```python
from build123d import *

# Parameters (mm, degrees)
F0_W     = 55.499
F0_H     = 37.5412
F0_W_2   = 52.959
F0_H_2   = 35.0012
F1_DEPTH = 1.27
F2_DEPTH = 7.62
F3_R     = 10.16


with BuildPart() as f1:
    # F0 (on Top) → F1 (new body)
    with BuildSketch(Plane.XY):
        with Locations((-37.199277, 3.972059)):
            Rectangle(F0_W, F0_H)
        with Locations((-37.199277, 3.972059)):
            Rectangle(F0_W_2, F0_H_2, mode=Mode.SUBTRACT)
        with Locations((-37.199277, 3.972059)):
            Rectangle(F0_W_2, F0_H_2)
    extrude(amount=F1_DEPTH)

    # F0 (on Top) → F2 (join)
    with BuildSketch(Plane.XY):
        with Locations((-37.199277, 3.972059)):
            Rectangle(F0_W, F0_H)
        with Locations((-37.199277, 3.972059)):
            Rectangle(F0_W_2, F0_H_2, mode=Mode.SUBTRACT)
    extrude(amount=F2_DEPTH)

    # F3
    f3_edges = [f1.edges().sort_by_distance(p)[0] for p in [
        (-64.948777, 22.742659, 3.81),
        (-63.678777, 21.472659, 4.445),
        (-10.719777, -13.528541, 4.445),
        (-9.449777, -14.798541, 3.81),
    ]]
    fillet(f3_edges, radius=F3_R)


solid = f1.part
```
The listing builds one solid part. Answer for the finished solid, in the listing's coordinates (mm). A direction names the side the tool comes from. Coordinates: 2 decimals unless noted, no trailing zeros. Loops run counter-clockwise (first coordinate to the right, second up) from the corner with the lowest first, then second, coordinate; pieces in that order, holes last. Notation, with made-up numbers: (81, 45) -> (121, 45) arc R28 cw to (121, 80) -> close; hole circle Ø8 at (78.5, -17). An arc over 180 degrees is marked (long way). Return JSON: item names as keys, results as strings. Group by question number.
(1) A cutting plane is placed at A-A on z = 3.5. Write down the section's boundary in (x, y).
(2) A cutting plane is placed at C-C on y = 9. Write down the section's boundary in (x, z), and give its area (3 significant figures).
(3) Given pin 1 Ø2 at (x, z) = (-18, 3.5) entering from -Y; pin 2 Ø10 at (x, y) = (-32.5, 16) entering from +Z, each flat-ended and moving along its own axis, determine where each tip first touches the part or whether it passes through.
(4) A cutting plane is placed at B-B on x = -44. Write down the section's boundary in (y, z).
(5) Determine the mould class of faces 3 (the flat face through (-64.949, -1, 4)), 4 (the flat face through (-10.72, 9, 4)), 5 (the flat face through (-43, -14.799, 4)), 6 (the flat face through (-9.45, 9, 4)) for opening direction X: released by +X, released by -X, zero draft, split by the parting line, or undercut.
(6) Find the intervals of material crossed by probe 1 along Y at (x, z) = (-32.5, 2.5); probe 2 along X at (y, z) = (2.5, 1.5); probe 3 along Z at (x, y) = (-13, 19.5), in increasing order. Write a range as from..to.
(7) Which of the six approach directions +Z, -Z, +X, -X, +Y, -Y give full straight-line access (tool end or side, diameter ignored) to faces 1 (the flat face through (-43, -13.529, 4)), 2 (the cylindrical face through (-12.347, -11.743, 3.863))?
The answers:
{
 "1": {"outline": "(-64.95, -14.8) -> (-19.61, -14.8) arc R10.16 ccw to (-9.45, -4.64) -> (-9.45, 22.74) -> (-54.79, 22.74) arc R10.16 ccw to (-64.95, 12.58) -> close; hole (-63.68, -13.53) -> (-20.88, -13.53) arc R10.16 ccw to (-10.72, -3.37) -> (-10.72, 21.47) -> (-53.52, 21.47) arc R10.16 ccw to (-63.68, 11.31) -> close"},
 "2": {"outline": "(-64.95, 0) -> (-9.45, 0) -> (-9.45, 7.62) -> (-10.72, 7.62) -> (-10.72, 1.27) -> (-63.68, 1.27) -> (-63.68, 7.62) -> (-64.95, 7.62) -> close", "area": "86.6 mm^2"},
 "3": {"pin 1": "stops at y = -14.78", "pin 2": "stops at z = 1.27"},
 "4": {"outline": "(-14.8, 0) -> (22.74, 0) -> (22.74, 7.62) -> (21.47, 7.62) -> (21.47, 1.27) -> (-13.53, 1.27) -> (-13.53, 7.62) -> (-14.8, 7.62) -> close"},
 "5": {"face 3": "released by -X", "face 4": "undercut", "face 5": "zero draft", "face 6": "released by +X"},
 "6": {"probe 1": "y = -14.8..-13.53, 21.47..22.74", "probe 2": "x = -64.95..-63.68, -10.72..-9.45", "probe 3": "z = 0..1.27"},
 "7": {"face 1": "+Z", "face 2": "+Z, -Z, +X, -Y"}
}
